For this review, take the finished solid that the model builds, in its own axes (mm). A direction names the side the tool comes from. Give positions to 0.01 mm unless a question says otherwise; leave off trailing zeros. Order: outer loops, then holes, each group sorted by start corner. A loop starts at its lowest first (then second) coordinate and runs counter-clockwise, first axis right, second up. Notation, with made-up numbers: (10.5, 4.5) -> (24.5, 4.5) arc R18 cw to (24.5, 34.5) -> close; hole circle Ø3 at (-4.5, 4). An arc over 180 degrees is marked (long way). Return JSON: item names as keys, results as strings. Group by question number.
1) Add section B-B (z = 2.85). Give the boundary of the cut face in (x, y).
2) Add section A-A (y = 14). Give the boundary of the cut face in (x, z), then the cut area to 3 significant figures.
3) Insertion check: P1, Ø1, axis at y = 7, z = 3, coming from the +X side; P2, Ø1.5, axis at x = 1, z = 2.5, coming from the +Y side; P3, Ø1.1, axis at y = 11.5, z = 5, coming from the -X side; P4, Ø8, axis at x = 10.5, y = 7, coming from the -Z side. Each pin has a flat end and moves straight along its axis. Give the tip position at first contact, or say it passes through.
4) For faces 4 (the face through (19, 20, 1)), 5 (the face through (20, 1.5, 5)), 6 (the face through (2, 10, 5)), 7 (the face through (17.5, 11, 3)), 8 (the face through (-0.5, 20, 1)), list the 3-axis set-ups (+Z, -Z, +X, -X, +Y, -Y) from which the entire face can be reached by the end or side of a thin tool; tool diameter is ignored.
5) To check wall thickness, follow line 1 along X through (y, z) = (4.5, 1.2); line 2 along X through (y, z) = (6, 5.15); line 3 along Y through (x, z) = (9.5, 1.65). State the ranges of each line that lie inside material, in increasing order.
6) The part is to be moulded in two halves that separate along Y. For faces 1 (the face through (22.25, 0.73, 5.01)), 2 (the face through (-0.5, 0.5, 1)), 3 (the face through (2.519, 22.285, 5.007)), say which applies: released by +Y, released by -Y, zero draft, split by the parting line, or undercut.
7) Add section C-C (x = 19). Give the boundary of the cut face in (y, z).
8) Add section D-D (y = 22.5). Give the boundary of the cut face in (x, z).
Autodesk Inventor part; units mm, degrees
ref_plane "YZ Plane" through (0, 0, 0) normal (1, 0, 0) x (0, 1, 0)
ref_plane "XZ Plane" through (0, 0, 0) normal (0, 1, 0) x (-1, 0, 0)
ref_plane "XY Plane" through (0, 0, 0) normal (0, 0, 1) x (1, 0, 0)
sketch "Skizze1" plane through (0, 0, 0) normal (0, 0, 1) x (1, 0, 0)
  line L0 (0, 0) -> (18.5, 0)
  line L1 (18.5, 0) -> (18.5, 20.5)
  line L2 (18.5, 20.5) -> (0, 20.5)
  line L3 (0, 20.5) -> (0, 0)
  dimension "d0" = 18.5
  dimension "d1" = 20.5
extrude "Extrusion1" add sketch "Skizze1" along normal blind 5.5
sketch "Skizze2" plane through (0, 20.5, 0) normal (0, 1, 0) x (1, 0, 0)
  line L0 (18.5, 0) -> (0, 0)
  line L1 (0, 0) -> (0, -5.5)
  line L2 (18.5, -5.5) -> (0, -5.5)
  line L3 (18.5, 0) -> (18.5, -5.5)
  line L4 (1, -1) -> (17.5, -1)
  line L5 (17.5, -1) -> (17.5, -4.5)
  line L6 (17.5, -4.5) -> (1, -4.5)
  line L7 (1, -4.5) -> (1, -1)
  line L8 (2, -4.5) -> (2, -5.5)
  line L9 (18.5, -5.5) -> (0, -5.5)
  line L10 (16.5, -4.5) -> (16.5, -5.5)
  line L11 (16.5, -1) -> (16.5, 0)
  line L12 (18.5, 0) -> (0, 0)
  line L13 (2, -1) -> (2, 0)
  point P0 (1, -2.75)
  point P1 (0, -2.75)
  point P2 (9.25, -1)
  point P3 (9.25, 0)
  point P4 (16.5, -5.5)
  point P5 (2, -5.5)
  point P6 (2, 0)
  point P7 (16.5, 0)
  dimension "d4" = 3.5
  dimension "d5" = 1
  dimension "d8" = 2
  dimension "d9" = 2
extrude "Extrusion2" cut sketch "Skizze2" against normal blind 19 contours L11 L4 L13 L0 | L4 L5 L6 L7 | L2 L8 L6 L10
sketch "Skizze3" plane through (0, 0, 0) normal (0, -1, 0) x (1, 0, 0)
  line L0 (0, 0) -> (18.5, 0)
  line L1 (18.5, 0) -> (18.5, 5.5)
  line L2 (0, 5.5) -> (18.5, 5.5)
  line L3 (0, 0) -> (0, 5.5)
  line L4 (0, 0) -> (0, 5.5)
  line L5 (0, 1) -> (-1, 1)
  line L6 (-1, 1) -> (0, 0)
  line L7 (18.5, 0) -> (18.5, 5.5)
  line L8 (18.5, 1) -> (19.5, 1)
  line L9 (19.5, 1) -> (18.5, 0)
  dimension "d10" = 1
  dimension "d11" = 1
extrude "Extrusion3" add sketch "Skizze3" against normal up to surface (20.5 mm away) contours L6 L5 L3 | L1 L8 L9
sketch "Skizze4" plane through (0, 0, 5.5) normal (0, 0, 1) x (1, 0, 0)
  line L0 (16.5, 20.5) -> (16.5, 1.5)
  line L1 (16.5, 1.5) -> (2, 1.5)
  line L2 (2, 1.5) -> (2, 20.5)
  line L3 (2, 20.5) -> (0, 20.5)
  line L4 (0, 20.5) -> (0, 0)
  line L5 (0, 0) -> (18.5, 0)
  line L6 (18.5, 0) -> (18.5, 20.5)
  line L7 (18.5, 20.5) -> (16.5, 20.5)
  line L8 (0, 20.5) -> (0, 0)
  line L9 (-1, 0) -> (-1, 20.5)
  line L10 (0, 19.5) -> (-1, 19.5)
  line L11 (-1, 19.5) -> (-1, 1)
  line L12 (-1, 1) -> (0, 1)
  line L13 (0, 1) -> (0, 19.5)
  line L14 (18.5, 0) -> (18.5, 20.5)
  line L15 (19.5, 0) -> (19.5, 20.5)
  line L16 (18.5, 19.5) -> (19.5, 19.5)
  line L17 (19.5, 19.5) -> (19.5, 1)
  line L18 (19.5, 1) -> (18.5, 1)
  line L19 (18.5, 1) -> (18.5, 19.5)
  line L20 (0, 20.5) -> (-1, 20.5)
  point P0 (0, 10.25)
  point P1 (18.5, 10.25)
  dimension "d14" = 1
extrude "Extrusion4" cut sketch "Skizze4" against normal through all contours L16 L15 L18 L6 | L4 L12 L9 L10
sketch "Skizze5" plane through (0, 0, 5.5) normal (0, 0, 1) x (1, 0, 0)
  line L0 (16.5, 20.5) -> (16.5, 1.5)
  line L1 (16.5, 1.5) -> (2, 1.5)
  line L2 (2, 1.5) -> (2, 20.5)
  line L3 (2, 20.5) -> (0, 20.5)
  line L4 (0, 20.5) -> (0, 0)
  line L5 (0, 0) -> (18.5, 0)
  line L6 (18.5, 0) -> (18.5, 20.5)
  line L7 (18.5, 20.5) -> (16.5, 20.5)
  line L8 (-3, 1.5) -> (21.5, 1.5)
  line L9 (21.5, 0) -> (-3, 0)
  arc A0 (-3, 1.5) -> (-3, 0) centre (-3, 0.75) ccw
  arc A1 (21.5, 0) -> (21.5, 1.5) centre (21.5, 0.75) ccw
  line L10 (-3, 17.0839) -> (-4.0261, 19.903)
  line L11 (-4.0261, 19.903) -> (9.25, 24.7351)
  line L12 (9.25, 24.7351) -> (22.5261, 19.903)
  line L13 (22.5261, 19.903) -> (21.5, 17.0839)
  line L14 (21.5, 17.0839) -> (9.25, 21.5425)
  line L15 (9.25, 21.5425) -> (-3, 17.0839)
  line L16 (16.5, 1.5) -> (2, 1.5)
  line L17 (-1, 17.8118) -> (-1, 1.5)
  line L18 (19.5, 1.5) -> (19.5, 17.8118)
  line L19 (2.513, 19.0905) -> (1.487, 21.9095) construction
  point P0 (9.25, 1.5)
  point P1 (18.5, 1.5)
  point P2 (0, 1.5)
  point P3 (9.25, 1.5)
  point P4 (2, 18.9037)
  point P5 (16.5, 18.9037)
  dimension "d18" = 3
  dimension "d31" = 20
  dimension "d32" = 3
  dimension "d33" = 1
extrude "Extrusion5" add sketch "Skizze5" against normal blind 1 contours L0 L14 L15 L2 L3 L4 L10 L11 L12 L13 L6 L7 | L8 L6 L5 L4 L1 | L14 L18 L8 L6 | L8 A1 L9 L6 | L8 L17 L15 L4 | L4 L9 A0 L8
equation "\"d9\" = d8"
properties part number "window_test"
Evaluation:
{
 "1": {"outline": "(0, 0) -> (18.5, 0) -> (18.5, 20.5) -> (17.5, 20.5) -> (17.5, 1.5) -> (1, 1.5) -> (1, 20.5) -> (0, 20.5) -> close"},
 "2": {"outline": "(-1, 4.5) -> (0, 4.5) -> (0, 0) -> (2, 0) -> (2, 1) -> (1, 1) -> (1, 4.5) -> (2, 4.5) -> (2, 5.5) -> (-1, 5.5) -> close; (16.5, 0) -> (18.5, 0) -> (18.5, 4.5) -> (19.5, 4.5) -> (19.5, 5.5) -> (16.5, 5.5) -> (16.5, 4.5) -> (17.5, 4.5) -> (17.5, 1) -> (16.5, 1) -> close", "area": "17.0 mm^2"},
 "3": {"P1": "x = 18.5", "P2": "y = 20.5", "P3": "x = -1", "P4": "through"},
 "4": {"face 4": "+X, +Y, -Y", "face 5": "+Z, -Z, +X", "face 6": "+Z, -Z", "face 7": "+Y", "face 8": "-X, +Y, -Y"},
 "5": {"line 1": "0 to 1, 17.5 to 18.5", "line 2": "-1 to 2, 16.5 to 19.5", "line 3": "0 to 1.5"},
 "6": {"face 1": "undercut", "face 2": "zero draft", "face 3": "released by +Y"},
 "7": {"outline": "(0, 0.5) -> (1, 0.5) -> (1, 1) -> (0, 1) -> close; (0, 4.5) -> (21.19, 4.5) -> (21.19, 5.5) -> (0, 5.5) -> close; (19.5, 0.5) -> (20.5, 0.5) -> (20.5, 1) -> (19.5, 1) -> close"},
 "8": {"outline": "(3.11, 4.5) -> (15.39, 4.5) -> (15.39, 5.5) -> (3.11, 5.5) -> close"}
}
